```python
from build123d import *

# Parameters (mm, degrees)
SKICA1_W     = 15
SKICA1_H     = 3
ZKOSIT1_SIZE = 0.5


with BuildPart() as part:
    # Skica1 → Otočit kolem osy1 (revolve)
    with BuildSketch(Plane.XY, mode=Mode.PRIVATE) as oto_it_kolem_osy1_sk:
        with Locations((7.5, 11.5)):
            Rectangle(SKICA1_W, SKICA1_H)
    revolve(oto_it_kolem_osy1_sk.sketch.rotate(Axis((0, 0, 0), (1, 0, 0)), 90), axis=Axis((0, 0, 0), (1, 0, 0)))

    # Zkosit1
    zkosit1_edges = [part.edges().sort_by_distance(p)[0] for p in [
        (0, 0, -10),
        (15, 0, -10),
        (15, 0, -13),
        (0, 0, -13),
    ]]
    chamfer(zkosit1_edges, length=ZKOSIT1_SIZE)


solid = part.part
```
Build history of the part. All positions in model axes, mm. Give positions to 0.01 mm unless a question says otherwise; leave off trailing zeros. Loops run counter-clockwise (first coordinate to the right, second up) from the corner with the lowest first, then second, coordinate; pieces in that order, holes last.
Item 1: Drill centre lines: line 1 (Y direction, x = 3.75, z = 0); line 2 (Y direction, x = 12.5, z = 7.25); line 3 (Z direction, x = 3, y = 5.75). Where is each one in solid material? Low to high.
Answers follow:
line 1: y = -13 to -10, 10 to 13
line 2: y = -10.79 to -6.89, 6.89 to 10.79
line 3: z = -11.66 to -8.18, 8.18 to 11.66
Item 2: Flat gauge pins, fed straight in: pin 1 (1.5 mm diameter, centred on x = 5, y = -5, fed in from -Z); pin 2 (6 mm diameter, centred on x = 8.5, z = 3.5, fed in from +Y); pin 3 (4 mm diameter, centred on x = 6.5, y = -6, fed in from +Z). Where does each tip first touch, or does it go through?
Answers follow:
pin 1: stops at z = -12.29
pin 2: stops at y = 12.99
pin 3: stops at z = 12.37
Item 3: Slice it at C-C, the plane x = 3.5. List the corners of the cut face in (y, z).
Answers follow:
outline: circle Ø26 at (0, 0); hole circle Ø20 at (0, 0)
Item 4: Slice it at A-A, the plane z = 0. List the corners of the cut face in (x, y), and give its area (3 significant figures).
Answers follow:
outline: (0, -12.5) - (0.5, -13) - (14.5, -13) - (15, -12.5) - (15, -10.5) - (14.5, -10) - (0.5, -10) - (0, -10.5) - close; (0, 10.5) - (0.5, 10) - (14.5, 10) - (15, 10.5) - (15, 12.5) - (14.5, 13) - (0.5, 13) - (0, 12.5) - close
area: 89.0 mm2
Item 5: Pull direction Z, two halves, no side cores. Call faces 1 (the face through (8, 0, -10)), 2 (the face through (7.598, 7.91, -10.316)): released by +Z, released by -Z, zero draft, split by the parting line, or undercut.
Answers follow:
face 1: undercut
face 2: split by the parting line
